For this review, take the finished solid that the model builds, in its own axes (mm). A direction names the side the tool comes from. Give positions to 0.01 mm unless a question says otherwise; leave off trailing zeros. Order: outer loops, then holes, each group sorted by start corner. A loop starts at its lowest first (then second) coordinate and runs counter-clockwise, first axis right, second up. Notation, with made-up numbers: (-14, 65) -> (-5, 65) arc R9 ccw to (-5, 76) -> close; hole circle Ø9 at (2, 38). An arc over 180 degrees is marked (long way). Return JSON: item names as keys, results as strings. Group by question number.
1) To check wall thickness, follow line 1 along Z through (x, y) = (9, -8); line 2 along Y through (x, z) = (-120, -13.5). State the ranges of each line that lie inside material, in increasing order.
2) Add section C-C (x = -12). Give the boundary of the cut face in (y, z) (3 decimals).
3) Add section A-A (z = 1). Give the boundary of the cut face in (x, y), then the cut area to 3 significant figures.
4) For faces 1 (the face through (2, 19.05, 0)), 2 (the face through (2, 16.51, 0)), list the 3-axis set-ups (+Z, -Z, +X, -X, +Y, -Y) from which the entire face can be reached by the end or side of a thin tool; tool diameter is ignored.
5) Add section B-B (y = -13). Give the boundary of the cut face in (x, z), then the cut area to 3 significant figures.
6) The part is to be moulded in two halves that separate along Y. For faces 3 (the face through (2, 0, 16.51)), 4 (the face through (2, 0, 19.05)), 5 (the face through (2, 0, -16.51)), 6 (the face through (-120.92, -0.27, -16.67)), say which applies: released by +Y, released by -Y, zero draft, split by the parting line, or undercut.
from build123d import *

# Parameters (mm, degrees)
EXTRUDE_THIN1_DEPTH     = 131.7625
CUT_EXTRUDE1_DEPTH      = 1
CUT_EXTRUDE1_DEPTH_BACK = 39.1
CUT_EXTRUDE2_DEPTH      = 1
CUT_EXTRUDE2_DEPTH_BACK = 39.1


with BuildPart() as part:
    # Sketch1 → Extrude-Thin1 (new body, symmetric)
    with BuildSketch(Plane(origin=(0, 0, 0), x_dir=(0, 0, -1), z_dir=(1, 0, 0))):
        with BuildLine():
            Line((-15.875, 19.05), (15.875, 19.05))
            ThreePointArc((15.875, 19.05), (18.12006403, 18.12006403), (19.05, 15.875))
            Line((19.05, 15.875), (19.05, -15.875))
            ThreePointArc((19.05, -15.875), (18.12006403, -18.12006403), (15.875, -19.05))
            Line((15.875, -19.05), (-15.875, -19.05))
            ThreePointArc((-15.875, -19.05), (-18.12006403, -18.12006403), (-19.05, -15.875))
            Line((-19.05, -15.875), (-19.05, 15.875))
            ThreePointArc((-19.05, 15.875), (-18.12006403, 18.12006403), (-15.875, 19.05))
        make_face()
        with BuildLine():
            Line((-15.875, 16.51), (15.875, 16.51))
            ThreePointArc((15.875, 16.51), (16.324012806, 16.324012806), (16.51, 15.875))
            Line((16.51, 15.875), (16.51, -15.875))
            ThreePointArc((16.51, -15.875), (16.324012806, -16.324012806), (15.875, -16.51))
            Line((15.875, -16.51), (-15.875, -16.51))
            ThreePointArc((-15.875, -16.51), (-16.324012806, -16.324012806), (-16.51, -15.875))
            Line((-16.51, -15.875), (-16.51, 15.875))
            ThreePointArc((-16.51, 15.875), (-16.324012806, 16.324012806), (-15.875, 16.51))
        make_face(mode=Mode.SUBTRACT)
    extrude(amount=EXTRUDE_THIN1_DEPTH, both=True)

    # Sketch2 → Cut-Extrude1 (cut, two sides)
    with BuildSketch(Plane.XY.offset(19.05)) as cut_extrude1_sk:
        Polygon((-403.027472584, -488.894714829), (-131.7625, -19.05), (-109.765454744, 19.05), (161.49951784, 488.894714829), (-778.189911818, 1031.424659996), (-1342.716902241, 53.635230339), align=None)
    extrude(amount=CUT_EXTRUDE1_DEPTH, mode=Mode.SUBTRACT)
    extrude(cut_extrude1_sk.sketch, amount=-CUT_EXTRUDE1_DEPTH_BACK, mode=Mode.SUBTRACT)

    # Sketch3 → Cut-Extrude2 (cut, two sides)
    with BuildSketch(Plane.XY.offset(19.05)) as cut_extrude2_sk:
        Polygon((403.027472584, -488.894714829), (131.7625, -19.05), (109.765454744, 19.05), (-161.49951784, 488.894714829), (778.189911818, 1031.424659996), (1342.716902241, 53.635230339), align=None)
    extrude(amount=CUT_EXTRUDE2_DEPTH, mode=Mode.SUBTRACT)
    extrude(cut_extrude2_sk.sketch, amount=-CUT_EXTRUDE2_DEPTH_BACK, mode=Mode.SUBTRACT)


solid = part.part
Evaluation:
{
 "1": {"line 1": "-19.05 to -16.51, 16.51 to 19.05", "line 2": "-19.05 to -16.51"},
 "2": {"outline": "(-19.05, -15.875) arc R3.175 ccw to (-15.875, -19.05) -> (15.875, -19.05) arc R3.175 ccw to (19.05, -15.875) -> (19.05, 15.875) arc R3.175 ccw to (15.875, 19.05) -> (-15.875, 19.05) arc R3.175 ccw to (-19.05, 15.875) -> close; hole (-16.51, -15.875) arc R0.635 ccw to (-15.875, -16.51) -> (15.875, -16.51) arc R0.635 ccw to (16.51, -15.875) -> (16.51, 15.875) arc R0.635 ccw to (15.875, 16.51) -> (-15.875, 16.51) arc R0.635 ccw to (-16.51, 15.875) -> close"},
 "3": {"outline": "(-131.76, -19.05) -> (131.76, -19.05) -> (130.3, -16.51) -> (-130.3, -16.51) -> close; (-111.23, 16.51) -> (111.23, 16.51) -> (109.77, 19.05) -> (-109.77, 19.05) -> close", "area": "1,230 mm^2"},
 "4": {"face 1": "+Z, -Z, +X, -X, +Y", "face 2": "+X, -X"},
 "5": {"outline": "(-128.27, -19.05) -> (128.27, -19.05) -> (128.27, -16.51) -> (-128.27, -16.51) -> close; (-128.27, 16.51) -> (128.27, 16.51) -> (128.27, 19.05) -> (-128.27, 19.05) -> close", "area": "1,300 mm^2"},
 "6": {"face 3": "undercut", "face 4": "zero draft", "face 5": "undercut", "face 6": "released by +Y"}
}
